Input: part model. Units: mm. Frame: model coordinates. Face numbers are marked on the shaded views. A direction names the side the tool comes from. Give positions to 0.01 mm unless a question says otherwise; leave off trailing zeros. Loops run counter-clockwise (first coordinate to the right, second up) from the corner with the lowest first, then second, coordinate; pieces in that order, holes last. Notation, with made-up numbers: M 82.5,48 L 128.5,48 A22 ccw 128.5,87 Z; hole C 55.5,-24.75 d1. An arc over 180 degrees is marked long. One line per item, written item: value. Start each with the question number.
(1) Section D-D on x = 3.25. Output: boundary loops of the cut face in (y, z).
(2) Section B-B on y = 13. Output: boundary loops of the cut face in (x, z).
(3) Section A-A on x = 0. Output: boundary loops of the cut face in (y, z).
(4) Section C-C on y = 20. Output: boundary loops of the cut face in (x, z), plus the area to 3 significant figures.
(5) Pin query (flat end, axial travel): P1, Ø1.7, axis at x = -0.5, z = -0.5, coming from the +Y side; P2, Ø1, axis at x = -2.5, z = 0, coming from the -Y side. Return the tip coordinate at first contact, or that it passes through.
(6) Ray query, line 1 along X through (y, z) = (17.5, 0); line 2 along Y through (x, z) = (1.5, 2.25); line 3 along Y through (x, z) = (3, 0.5). Return the intervals inside material, ascending. Write a range as from..to.
(7) Access query for the marked faces 1, 2, 3, 4 and 5. Directions: +Z, -Z, +X, -X, +Y, -Y. A direction counts if a zero-diameter tool reaches every point of the face in a straight line with its end or side. Return the directions, or none.
(8) Pull-direction query (Y, two-part tool) for the marked faces 6, 7 and 8; classes: released by +Y, released by -Y, zero draft, split by the parting line, or undercut.
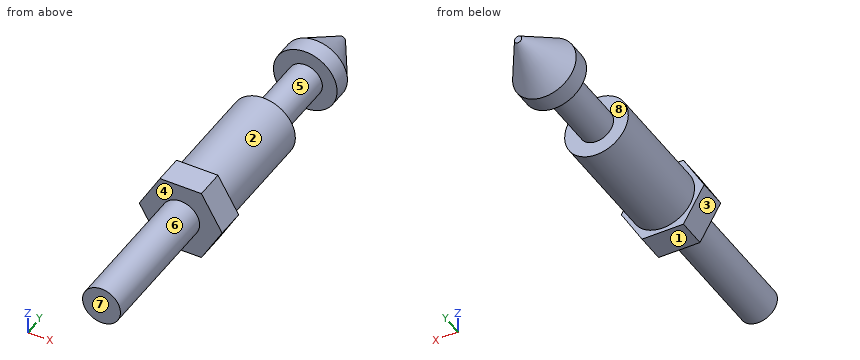
```python
from build123d import *

# Parameters (mm, degrees)
BOSS_EXTRUDE1_DEPTH = 2.54


with BuildPart() as part:
    # Sketch1 → Revolve1 (revolve)
    with BuildSketch(Plane.XY, mode=Mode.PRIVATE) as revolve1_sk:
        Polygon((0, 0), (1.6637, 0), (1.6637, 12.1412), (2.794, 12.1412), (2.794, 24.8412), (1.4986, 24.8412), (1.4986, 31.242), (2.794, 31.242), (2.794, 32.8295), (0.3175, 36.8554), (0, 36.8554), align=None)
    revolve(revolve1_sk.sketch.rotate(Axis((0, 0, 0), (0, 1, 0)), 90), axis=Axis((0, 0, 0), (0, 1, 0)))  # turned: the seam where the file's is

    # Sketch2 → Boss-Extrude1 (add)
    with BuildSketch(Plane.XZ.offset(-12.1412)):
        Polygon((3.636844816, 0), (1.818422408, 3.1496), (-1.818422408, 3.1496), (-3.636844816, 0), (-1.818422408, -3.1496), (1.818422408, -3.1496), align=None)
    extrude(amount=-BOSS_EXTRUDE1_DEPTH)


solid = part.part
```
Output values:
1. outline: M 12.14,-0.67 L 14.68,-0.67 L 14.68,0.67 L 12.14,0.67 Z
2. outline: M -3.64,0 L -1.82,-3.15 L 1.82,-3.15 L 3.64,0 L 1.82,3.15 L -1.82,3.15 Z
3. outline: M 0,-1.66 L 12.14,-1.66 L 12.14,-3.15 L 14.68,-3.15 L 14.68,-2.79 L 24.84,-2.79 L 24.84,-1.5 L 31.24,-1.5 L 31.24,-2.79 L 32.83,-2.79 L 36.86,-0.32 L 36.86,0.32 L 32.83,2.79 L 31.24,2.79 L 31.24,1.5 L 24.84,1.5 L 24.84,2.79 L 14.68,2.79 L 14.68,3.15 L 12.14,3.15 L 12.14,1.66 L 0,1.66 Z
4. outline: C 0,0 d5.59
4. area: 24.5 mm²
5. P1: stops at y = 36.86
5. P2: stops at y = 12.14
6. line 1: x = -2.79..2.79
6. line 2: y = 12.14..24.84, 31.24..32.98
6. line 3: y = 12.14..14.68
7. face 1: -Z, +X, -X, +Y, -Y
7. face 2: +Y
7. face 3: -Z, -X, +Y, -Y
7. face 4: -Y
7. face 5: none
8. face 6: zero draft
8. face 7: released by -Y
8. face 8: undercut
